Autodesk Inventor part; units mm, degrees
ref_plane "YZ Plane" through (0, 0, 0) normal (1, 0, 0) x (0, 1, 0)
ref_plane "XZ Plane" through (0, 0, 0) normal (0, 1, 0) x (-1, 0, 0)
ref_plane "XY Plane" through (0, 0, 0) normal (0, 0, 1) x (1, 0, 0)
sketch "Sketch1" plane through (0, 0, 0) normal (0, 0, 1) x (1, 0, 0)
  line L0 (-62, 15) -> (62, 15)
  line L1 (62, 15) -> (62, -15)
  line L2 (62, -15) -> (-62, -15)
  line L3 (-62, -15) -> (-62, 15)
  line L4 (-62, 15) -> (62, -15) construction
  line L5 (62, 15) -> (-62, -15) construction
  point P0 (0, 0)
  dimension "d0" = 124
  dimension "d1" = 30
extrude "Extrusion1" add sketch "Sketch1" along normal blind 3
sketch "Sketch3" plane through (0, 0, 3) normal (0, 0, 1) x (1, 0, 0)
  line L0 (62, 15) -> (-62, 15)
  line L1 (-62, -15) -> (62, -15)
  arc A0 (-62, -15) -> (-52, -15) centre (-57, -15) ccw
  line L2 (-62, -15) -> (-52, -15)
  point P0 (0, 0)
extrude "Extrusion3" add sketch "Sketch3" against normal blind 3
mirror "Mirror2" about plane through (0, 0, 0) normal (1, 0, 0) of "Extrusion3"
fillet "Fillet1" radius 2 1 edges at (-62, 15, 1.5)
fillet "Fillet2" radius 2 1 edges at (62, 15, 1.5)
sketch "Sketch5" plane through (0, 0, 3) normal (0, 0, 1) x (1, 0, 0)
  line L0 (-58.91, 12.96) -> (-56.09, 12.96)
  line L1 (-56.09, 12.96) -> (-56.09, 8.04)
  line L2 (-56.09, 8.04) -> (-58.91, 8.04)
  line L3 (-58.91, 8.04) -> (-58.91, 12.96)
  line L4 (-58.91, 12.96) -> (-56.09, 8.04) construction
  line L5 (-56.09, 12.96) -> (-58.91, 8.04) construction
  line L6 (60, 15) -> (-60, 15)
  line L7 (-58.91, -8.04) -> (-56.09, -8.04)
  line L8 (-56.09, -8.04) -> (-56.09, -12.96)
  line L9 (-56.09, -12.96) -> (-58.91, -12.96)
  line L10 (-58.91, -12.96) -> (-58.91, -8.04)
  line L11 (-58.91, -8.04) -> (-56.09, -12.96) construction
  line L12 (-56.09, -8.04) -> (-58.91, -12.96) construction
  line L13 (-52, -15) -> (52, -15)
  point P0 (0, 0)
  point P1 (-57.5, 10.5)
  point P2 (-57.5, -10.5)
  point P3 (-57.5, -10.5)
  point P4 (-57.5, 10.5)
  dimension "d31" = 2.82
  dimension "d32" = 4.92
  dimension "d33" = 57.5
  dimension "d34" = 4.5
  dimension "d35" = 4.5
  dimension "d4" = 3
  dimension "d5" = 5
  dimension "d6" = 56
  dimension "d7" = 2
  dimension "d10" = 5
  dimension "d11" = 2
extrude "Extrusion5" cut sketch "Sketch5" against normal through all
mirror "Mirror3" about plane through (0, 0, 0) normal (1, 0, 0) of "Extrusion5"
equation "\"kerf\" = 0.13"
properties part number "BackPanel" material "Acrylic, Clear"
Build history of the part. All positions in model axes, mm. A direction names the side the tool comes from. Round coordinates to 2 decimals unless told otherwise and drop trailing zeros. Write each loop counter-clockwise with the first axis right and the second up, starting at its lowest first coordinate (ties: lowest second). Pieces come first, ordered by that corner, then holes. Notation, with made-up numbers: (80, 85) -> (136, 85) arc R12 ccw to (136, 93) -> close; hole circle Ø9 at (62.25, 65). An arc over 180 degrees is marked (long way). Use one line per item in the form item = value.
Q1. Drill centre lines: L1, parallel to X at y = -12, z = 0.6; L2, parallel to Y at x = -3.5, z = 2; L3, parallel to X at y = -16, z = 0.6. Where is each one in solid material? Low to high.
Conclusion:
L1 = -62 to -58.91, -56.09 to 56.09, 58.91 to 62
L2 = -15 to 15
L3 = -61.9 to -52.1, 52.1 to 61.9
Q2. Band-saw the part on A-A, the plane y = -11.5. Write the cut outline in (x, z).
Conclusion:
outline = (-62, 0) -> (-58.91, 0) -> (-58.91, 3) -> (-62, 3) -> close; (-56.09, 0) -> (56.09, 0) -> (56.09, 3) -> (-56.09, 3) -> close; (58.91, 0) -> (62, 0) -> (62, 3) -> (58.91, 3) -> close
Q3. Band-saw the part on C-C, the plane x = -24. Write the cut outline in (y, z).
Conclusion:
outline = (-15, 0) -> (15, 0) -> (15, 3) -> (-15, 3) -> close
Q4. Tool access for faces 5 (the flat face through (-58.91, -11, 2)), 6 (the cylindrical face through (-57, -20, 2)): list every direction of +Z, -Z, +X, -X, +Y, -Y with a clear straight run to the whole face (end or side of a thin tool).
Conclusion:
face_5 = +Z, -Z
face_6 = +Z, -Z, -Y
Q5. Band-saw the part on B-B, the plane z = 2.35. Write the cut outline in (x, y).
Conclusion:
outline = (-62, -15) arc R5 ccw to (-52, -15) -> (52, -15) arc R5 ccw to (62, -15) -> (62, 13) arc R2 ccw to (60, 15) -> (-60, 15) arc R2 ccw to (-62, 13) -> close; hole (-58.91, -12.96) -> (-56.09, -12.96) -> (-56.09, -8.04) -> (-58.91, -8.04) -> close; hole (-58.91, 8.04) -> (-56.09, 8.04) -> (-56.09, 12.96) -> (-58.91, 12.96) -> close; hole (56.09, -12.96) -> (58.91, -12.96) -> (58.91, -8.04) -> (56.09, -8.04) -> close; hole (56.09, 8.04) -> (58.91, 8.04) -> (58.91, 12.96) -> (56.09, 12.96) -> close
Q6. Two-plate mould, pull along X, no slides. Class faces 1 (the flat face through (-1, -2, 0)), 2 (the flat face through (58.91, -10, 2)), 3 (the cylindrical face through (-61.4, 14.43, 1.52)), 4 (the flat face through (-57, 8.04, 2)): released by +X, released by -X, zero draft, split by the parting line, or undercut.
Conclusion:
face_1 = zero draft
face_2 = undercut
face_3 = released by -X
face_4 = undercut
